Here's how the part is built. I have some questions about the finished solid (model axes, mm). Face numbers are marked on the shaded views. A direction names the side the tool comes from. Coordinates: 2 decimals unless noted, no trailing zeros. Loops run counter-clockwise (first coordinate to the right, second up) from the corner with the lowest first, then second, coordinate; pieces in that order, holes last. Notation, with made-up numbers: (81.25, 46.25) -> (139.25, 46.25) arc R34 cw to (139.25, 84.25) -> close; hole circle Ø4 at (88.25, 40.25). An arc over 180 degrees is marked (long way). Answer as a JSON object with one key per item and string values. Group by question number.
Q1. On a 3-axis mill with a long thin cutter (end or side, diameter ignored), from which of +Z, -Z, +X, -X, +Y, -Y can I reach the whole of each face in a straight line? I mean the marked faces 1 and 2. Say none if no direction works.
Q2. I'm going to push flat-ended pins straight in: pin 1 (6 mm diameter, centred on x = 22.5, z = -12, fed in from +Y); pin 2 (5 mm diameter, centred on x = 53.5, z = -9, fed in from -Y). Where does each tip first touch, or does it pass through?
Q3. I want a section at C-C on z = 21. Write out the boundary of the cut face in (x, y), then the cut area to 3 significant figures.
Q4. I want a section at A-A on y = -16. Write out the boundary of the cut face in (x, z).
Q5. I need wall thicknesses on line 1 (X direction, y = -17, z = 29.5); line 2 (Z direction, x = 10, y = -19.25); line 3 (Y direction, x = -21, z = -36.5). Which ranges of each line are inside material? Lowest first, please.
Q6. Thinking about a two-plate mould opening in Z: for the marked faces 3, 4, 5 and 6, which applies, released by +Z, released by -Z, zero draft, split by the parting line, or undercut?
Q7. I want a section at B-B on x = 32. Write out the boundary of the cut face in (y, z).
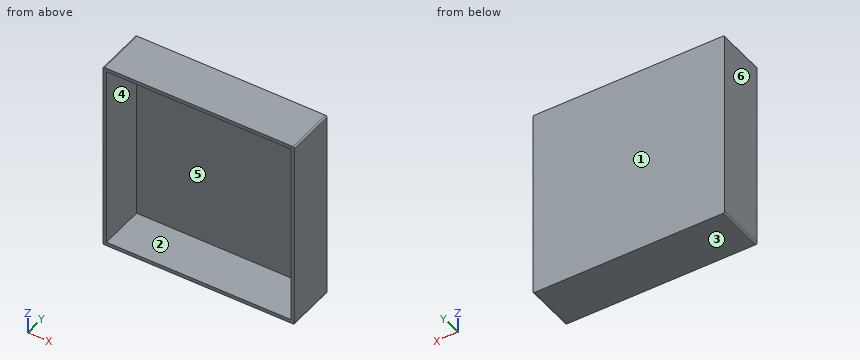
```python
from build123d import *

# Parameters (mm, degrees)
F0_W     = 105
F0_H     = 105
F1_DEPTH = 27
F2_T     = -2
F3_R     = 1


with BuildPart() as f1:
    # F0 (on Front) → F1 (new body)
    with BuildSketch(Plane.XZ):
        with Locations((14.582235, 5.405142)):
            Rectangle(F0_W, F0_H)
    extrude(amount=F1_DEPTH)

    # F2
    f2_openings = [f1.faces().sort_by_distance(p)[0] for p in [
        (14.582235, -27, 5.405142),
    ]]
    offset(amount=F2_T, openings=f2_openings)

    # F3
    f3_edges = [f1.edges().sort_by_distance(p)[0] for p in [
        (67.082235, -13.5, 57.905142),
        (67.082235, -13.5, -47.094858),
        (-37.917765, -13.5, 57.905142),
        (-37.917765, -13.5, -47.094858),
    ]]
    fillet(f3_edges, radius=F3_R)


solid = f1.part
```
Result set:
{
 "1": {"face 1": "+Z, -Z, +X, -X, +Y", "face 2": "-Y"},
 "2": {"pin 1": "stops at y = 0", "pin 2": "stops at y = -2"},
 "3": {"outline": "(-37.92, -27) -> (-35.92, -27) -> (-35.92, -2) -> (65.08, -2) -> (65.08, -27) -> (67.08, -27) -> (67.08, 0) -> (-37.92, 0) -> close", "area": "310 mm²"},
 "4": {"outline": "(-37.92, -46.09) arc R1 ccw to (-36.92, -47.09) -> (66.08, -47.09) arc R1 ccw to (67.08, -46.09) -> (67.08, 56.91) arc R1 ccw to (66.08, 57.91) -> (-36.92, 57.91) arc R1 ccw to (-37.92, 56.91) -> close; hole (-35.92, -45.09) -> (65.08, -45.09) -> (65.08, 55.91) -> (-35.92, 55.91) -> close"},
 "5": {"line 1": "x = -37.92 to -35.92, 65.08 to 67.08", "line 2": "z = -47.09 to -45.09, 55.91 to 57.91", "line 3": "y = -2 to 0"},
 "6": {"face 3": "released by -Z", "face 4": "undercut", "face 5": "undercut", "face 6": "zero draft"},
 "7": {"outline": "(-27, -47.09) -> (0, -47.09) -> (0, 57.91) -> (-27, 57.91) -> (-27, 55.91) -> (-2, 55.91) -> (-2, -45.09) -> (-27, -45.09) -> close"}
}
